The listing builds one solid part. Answer for the finished solid, in the listing's coordinates (mm). Coordinates: 2 decimals unless noted, no trailing zeros. Order: outer loops, then holes, each group sorted by start corner. A loop starts at its lowest first (then second) coordinate and runs counter-clockwise, first axis right, second up. Notation, with made-up numbers: (26.25, 79) -> (61.25, 79) arc R19 ccw to (61.25, 90) -> close; hole circle Ø3 at (2, -26.75). An arc over 180 degrees is marked (long way). Return JSON: item names as keys, results as strings.
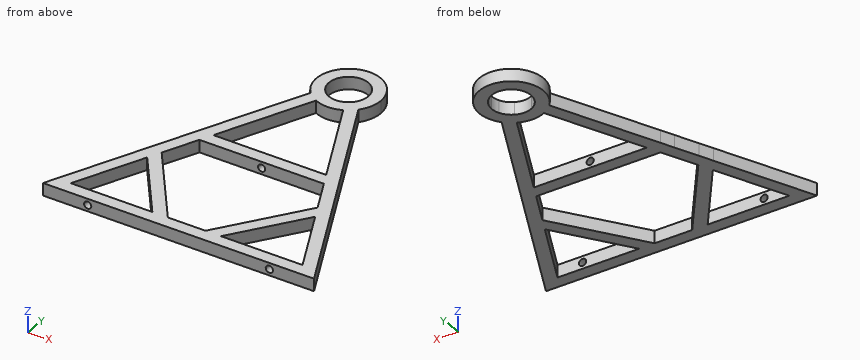
from build123d import *

# Parameters (mm, degrees)
F1_DEPTH = 7
F2_R     = 2
F3_DEPTH = 8
F4_R     = 2
F5_DEPTH = 8


# Not quite as in the source:
# - a feature names something its author has since deleted; it is built from what else it names


with BuildPart() as f1:
    # F0 (on Top) → F1 (new body)
    with BuildSketch(Plane.XY):
        with BuildLine():
            ThreePointArc((9.930189374, -4.7319487525), (7.7456068538, -7.8106065364), (4.6488008791, -9.9693856574))
            Line((4.6488008791, -9.9693856574), (7.6071287113, -16.3135401667))
            ThreePointArc((7.6071287113, -16.3135401667), (10.6923318533, -14.4801256741), (13.352485528, -12.0710865387))
            Line((13.352485528, -12.0710865387), (9.930189374, -4.7319487525))
        make_face()
        with BuildLine():
            Line((7.6071287113, -16.3135401667), (4.6488008791, -9.9693856574))
            ThreePointArc((4.6488008791, -9.9693856574), (0, -11), (-4.6488008791, -9.9693856574))
            Line((-4.6488008791, -9.9693856574), (-7.6071287113, -16.3135401667))
            ThreePointArc((-7.6071287113, -16.3135401667), (0, -18), (7.6071287113, -16.3135401667))
        make_face()
        with BuildLine():
            Line((-7.6071287113, -16.3135401667), (-4.6488008791, -9.9693856574))
            ThreePointArc((-4.6488008791, -9.9693856574), (-7.7456068538, -7.8106065364), (-9.930189374, -4.7319487525))
            Line((-9.930189374, -4.7319487525), (-13.352485528, -12.0710865387))
            ThreePointArc((-13.352485528, -12.0710865387), (-10.6923318533, -14.4801256741), (-7.6071287113, -16.3135401667))
        make_face()
        with BuildLine():
            ThreePointArc((13.352485528, -12.0710865387), (10.6923318533, -14.4801256741), (7.6071287113, -16.3135401667))
            Line((7.6071287113, -16.3135401667), (31.5509050579, -67.6611342449))
            Line((31.5509050579, -67.6611342449), (39.2745504906, -67.6611342449))
            Line((39.2745504906, -67.6611342449), (13.352485528, -12.0710865387))
        make_face()
        with BuildLine():
            ThreePointArc((11, 0), (10.7292143961, -2.4256872104), (9.930189374, -4.7319487525))
            Line((9.930189374, -4.7319487525), (13.352485528, -12.0710865387))
            ThreePointArc((13.352485528, -12.0710865387), (16.7979870744, -6.4674284107), (18, 0))
            ThreePointArc((18, 0), (-6.4674284107, 16.7979870744), (-13.352485528, -12.0710865387))
            Line((-13.352485528, -12.0710865387), (-9.930189374, -4.7319487525))
            ThreePointArc((-9.930189374, -4.7319487525), (-2.4256872104, 10.7292143961), (11, 0))
        make_face()
        with BuildLine():
            Line((-31.5509050579, -67.6611342449), (-7.6071287113, -16.3135401667))
            ThreePointArc((-7.6071287113, -16.3135401667), (-10.6923318533, -14.4801256741), (-13.352485528, -12.0710865387))
            Line((-13.352485528, -12.0710865387), (-39.2745504906, -67.6611342449))
            Line((-39.2745504906, -67.6611342449), (-31.5509050579, -67.6611342449))
        make_face()
        Polygon((39.2745504906, -67.6611342449), (31.5509050579, -67.6611342449), (34.8150586649, -74.6611342449), (42.5387040977, -74.6611342449), align=None)
        Polygon((34.8150586649, -74.6611342449), (31.5509050579, -67.6611342449), (-31.5509050579, -67.6611342449), (-34.8150586649, -74.6611342449), align=None)
        Polygon((-34.8150586649, -74.6611342449), (-31.5509050579, -67.6611342449), (-39.2745504906, -67.6611342449), (-42.5387040977, -74.6611342449), align=None)
        Polygon((42.5387040977, -74.6611342449), (34.8150586649, -74.6611342449), (43.6188979632, -93.5410285471), (48.3261309802, -87.0723112465), align=None)
        Polygon((-43.6188979632, -93.5410285471), (-34.8150586649, -74.6611342449), (-42.5387040977, -74.6611342449), (-48.3261309802, -87.0723112465), align=None)
        Polygon((48.3261309802, -87.0723112465), (43.6188979632, -93.5410285471), (46.9999060281, -100.7916237405), (51.7071390451, -94.3229064398), align=None)
        Polygon((46.9999060281, -100.7916237405), (43.6188979632, -93.5410285471), (10.5389814088, -138.9997147322), (19.1961886798, -138.9997147322), align=None)
        Polygon((-10.5389814088, -138.9997147322), (-43.6188979632, -93.5410285471), (-46.9999060281, -100.7916237405), (-19.1961886798, -138.9997147322), align=None)
        Polygon((-46.9999060281, -100.7916237405), (-43.6188979632, -93.5410285471), (-48.3261309802, -87.0723112465), (-51.7071390451, -94.3229064398), align=None)
        Polygon((51.7071390451, -94.3229064398), (46.9999060281, -100.7916237405), (64.816631461, -138.9997147322), (19.1961886798, -138.9997147322), (14.1023455596, -145.9997147322), (75.8044305008, -145.9997147322), align=None)
        Polygon((19.1961886798, -138.9997147322), (10.5389814088, -138.9997147322), (5.4451382885, -145.9997147322), (14.1023455596, -145.9997147322), align=None)
        Polygon((5.4451382885, -145.9997147322), (10.5389814088, -138.9997147322), (-10.5389814088, -138.9997147322), (-5.4451382885, -145.9997147322), align=None)
        Polygon((-64.816631461, -138.9997147322), (-46.9999060281, -100.7916237405), (-51.7071390451, -94.3229064398), (-75.8044305008, -145.9997147322), (-14.1023455596, -145.9997147322), (-19.1961886798, -138.9997147322), align=None)
        Polygon((-5.4451382885, -145.9997147322), (-10.5389814088, -138.9997147322), (-19.1961886798, -138.9997147322), (-14.1023455596, -145.9997147322), align=None)
    extrude(amount=F1_DEPTH)

    # F2 (on face) → F3 (cut)
    with BuildSketch(Plane(origin=(0, -67.6611342449, 0), x_dir=(-1, 0, 0), z_dir=(0, 1, 0))):
        with Locations((0, 3.5)):
            Circle(F2_R)
    extrude(amount=-F3_DEPTH, mode=Mode.SUBTRACT)

    # F4 (on face) → F5 (cut)
    with BuildSketch(Plane.XZ.offset(145.9997147322)):
        with Locations((-50.8044305008, 3.5)):
            Circle(F4_R)
        with Locations((50.8044305008, 3.5)):
            Circle(F4_R)
    extrude(amount=-F5_DEPTH, mode=Mode.SUBTRACT)


solid = f1.part
1. Consider line 1 (Y direction, x = 0, z = 1.75); line 2 (Y direction, x = 0, z = 5.75); line 3 (Y direction, x = 25.5, z = 1). Determine where each line is inside the solid, lowest interval first. Write a range as from..to.
Answer block:
{"line 1": "y = -146..-139, -18..-11, 11..18", "line 2": "y = -146..-139, -74.66..-67.66, -18..-11, 11..18", "line 3": "y = -146..-139, -130.34..-118.44, -74.66..-67.66, -54.68..-38.12"}
2. The part is cut by section B-B on y = -123. Give the vertices of the cut face in (x, z), and give its area (3 significant figures).
Answer block:
{"outline": "(-65.08, 0) -> (-57.36, 0) -> (-57.36, 7) -> (-65.08, 7) -> close; (-30.84, 0) -> (-22.18, 0) -> (-22.18, 7) -> (-30.84, 7) -> close; (22.18, 0) -> (30.84, 0) -> (30.84, 7) -> (22.18, 7) -> close; (57.36, 0) -> (65.08, 0) -> (65.08, 7) -> (57.36, 7) -> close", "area": "229 mm2"}
3. The part is cut by section C-C on x = 63. Give the vertices of the cut face in (y, z), and give its area (3 significant figures).
Answer block:
{"outline": "(-146, 0) -> (-139, 0) -> (-139, 7) -> (-146, 7) -> close; (-135.1, 0) -> (-118.54, 0) -> (-118.54, 7) -> (-135.1, 7) -> close", "area": "165 mm2"}
4. The part is cut by section A-A on x = 0. Give the vertices of the cut face in (y, z), and give its area (3 significant figures).
Answer block:
{"outline": "(-146, 0) -> (-139, 0) -> (-139, 7) -> (-146, 7) -> close; (-74.66, 0) -> (-67.66, 0) -> (-67.66, 1.5) -> (-74.66, 1.5) -> close; (-74.66, 5.5) -> (-67.66, 5.5) -> (-67.66, 7) -> (-74.66, 7) -> close; (-18, 0) -> (-11, 0) -> (-11, 7) -> (-18, 7) -> close; (11, 0) -> (18, 0) -> (18, 7) -> (11, 7) -> close", "area": "168 mm2"}
5. The part is cut by section D-D on z = 3.5. Give the number of separate pieces and of enclosed holes in the cut face, and give its area (3 significant figures).
Answer block:
{"separate pieces": "1", "enclosed holes": "2", "area": "4,710 mm2"}
6. Each of these flat-tipped pins is pushed along its axis until it touches: pin 1 Ø3 at (x, z) = (-50.8, 3.5) entering from +Y; pin 2 Ø2 at (x, z) = (-8.5, 2.5) entering from +Y; pin 3 Ø3 at (y, z) = (-100.5, 1) entering from -X. Where does it stop, or does it pass through?
Answer block:
{"pin 1": "stops at y = -89.16", "pin 2": "stops at y = 16.36", "pin 3": "stops at x = -55.29"}
